Here's how the part is built. I have some questions about the finished solid (model axes, mm). Face numbers are marked on the shaded views. Round coordinates to 2 decimals unless told otherwise and drop trailing zeros. Loops run counter-clockwise (first coordinate to the right, second up) from the corner with the lowest first, then second, coordinate; pieces in that order, holes last. Notation, with made-up numbers: M -9,71.25 L 44,71.25 A21 cw 44,79.25 Z; hole C -27,70 d3. An arc over 180 degrees is marked long. Use a Markdown table: item, result.
from build123d import *

# Parameters (mm, degrees)
SKETCH1_R           = 101.6
BOSS_EXTRUDE1_DEPTH = 254
SHELL1_T            = -2.54
SKETCH2_R           = 12.7
CUT_EXTRUDE1_DEPTH  = 254


with BuildPart() as part:
    # Sketch1 → Boss-Extrude1 (new body)
    with BuildSketch(Plane.XY):
        Circle(SKETCH1_R)
    extrude(amount=BOSS_EXTRUDE1_DEPTH)

    # Shell1
    shell1_openings = [part.faces().sort_by_distance(p)[0] for p in [
        (0, 0, 254),
    ]]
    offset(amount=SHELL1_T, openings=shell1_openings, kind=Kind.INTERSECTION)

    # Sketch2 → Cut-Extrude1 (cut)
    with BuildSketch(Plane.XY.offset(2.54)):
        Circle(SKETCH2_R)
    extrude(amount=-CUT_EXTRUDE1_DEPTH, mode=Mode.SUBTRACT)


solid = part.part
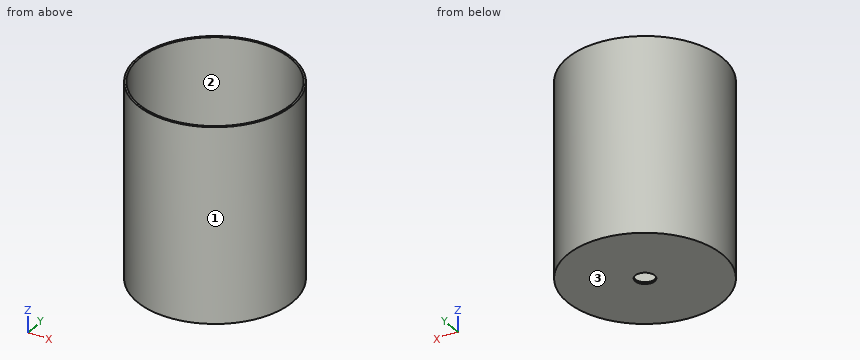
1. I need wall thicknesses on probe 1 along Y at (x, z) = (0, 0.8); probe 2 along Y at (x, z) = (0, 158.5); probe 3 along X at (y, z) = (-65.5, 60). Which ranges of each line are inside material? Lowest first, please. Write a range as from..to.
Answer sheet:
| item | result |
|---|---|
| probe 1 | -101.6..-12.7, 12.7..101.6 |
| probe 2 | -101.6..-99.06, 99.06..101.6 |
| probe 3 | -77.67..-74.31, 74.31..77.67 |
2. We'd pull the mould along Y, two halves only. Please class the marked faces 1, 2 and 3: +Y half, -Y half, draft (parallel to the pull), parting line (faces both ways), or undercut.
Answer sheet:
| item | result |
|---|---|
| face 1 | parting line |
| face 2 | undercut |
| face 3 | draft |
3. Imagine slicing it at D-D, the plane y = 49. Write out the boundary of the cut face in (x, z).
Answer sheet:
| item | result |
|---|---|
| outline | M -89,0 L 89,0 L 89,254 L 86.09,254 L 86.09,2.54 L -86.09,2.54 L -86.09,254 L -89,254 Z |
4. Imagine slicing it at A-A, the plane x = 0. Write out the boundary of the cut face in (y, z).
Answer sheet:
| item | result |
|---|---|
| outline | M -101.6,0 L -12.7,0 L -12.7,2.54 L -99.06,2.54 L -99.06,254 L -101.6,254 Z; M 12.7,0 L 101.6,0 L 101.6,254 L 99.06,254 L 99.06,2.54 L 12.7,2.54 Z |
5. For pin 1 Ø8 at (x, z) = (47.5, 159) entering from +Y; pin 2 Ø1 at (x, z) = (-75.5, 42.5) entering from -Y; pin 3 Ø10 at (y, z) = (-52, 134.5) entering from -X, each with a flat end and sliding along its axis, tell me the tip position at first contact or that it passes through.
Answer sheet:
| item | result |
|---|---|
| pin 1 | y = 91.82 |
| pin 2 | y = -68.54 |
| pin 3 | x = -90.08 |
6. Imagine slicing it at C-C, the plane x = -87.5. Write out the boundary of the cut face in (y, z).
Answer sheet:
| item | result |
|---|---|
| outline | M -51.64,0 L 51.64,0 L 51.64,254 L 46.44,254 L 46.44,2.54 L -46.44,2.54 L -46.44,254 L -51.64,254 Z |
